Work out the finished part from the listing and answer in its coordinate system (mm). Give positions to 0.01 mm unless a question says otherwise; leave off trailing zeros. Loops run counter-clockwise (first coordinate to the right, second up) from the corner with the lowest first, then second, coordinate; pieces in that order, holes last.
```python
from build123d import *

# Parameters (mm, degrees)
EXTRUDE1_DEPTH     = 3.175
SKETCH4_R          = 3.772
EXTRUDE3_DEPTH     = 1.27
SKETCH6_R          = 3
CUT_EXTRUDE1_DEPTH = 181.936091825


with BuildPart() as part:
    # Sketch1 → Extrude1 (new body)
    with BuildSketch(Plane.XY):
        with BuildLine():
            Line((104.316218765, 133.220465896), (119.791106556, 133.220465896))
            ThreePointArc((119.791106556, 133.220465896), (122.35366266, 126.720465896), (119.791106556, 120.220465896))
            Line((119.791106556, 120.220465896), (104.316218765, 120.220465896))
            ThreePointArc((104.316218765, 120.220465896), (101.75366266, 126.720465896), (104.316218765, 133.220465896))
        make_face()
    extrude(amount=EXTRUDE1_DEPTH)

    # Sketch4 → Extrude3 (add)
    with BuildSketch(Plane.XY.offset(3.175)):
        with Locations((117.35366266, 126.720465896)):
            Circle(SKETCH4_R)
    extrude(amount=EXTRUDE3_DEPTH)

    # Sketch6 → Cut-Extrude1 (cut, through all)
    with BuildSketch(Plane(origin=(0, 0, 0), x_dir=(-1, 0, 0), z_dir=(0, 0, -1))):
        with Locations((-117.35366266, 126.720465896)):
            Circle(SKETCH6_R)
    extrude(amount=-CUT_EXTRUDE1_DEPTH, mode=Mode.SUBTRACT)


solid = part.part
```
Q1. Section D-D on x = 107.5 is taken. Give the vertices of the cut face in (y, z) (3 decimals), plus the area to 3 significant figures.
Q2. Section B-B on y = 126.25 is taken. Give the vertices of the cut face in (x, z) (3 decimals).
Q3. Section C-C on z = 1 is taken. Give the vertices of the cut face in (x, y) (3 decimals), plus the area to 3 significant figures.
Q4. Determine the mould class of faces 1 (the face through (122.353, 126.821, 1.565)), 2 (the face through (120.951, 127.853, 3.801)), 3 (the face through (112, 133.22, 2)), 4 (the face through (114.49, 127.62, 2.19)) for opening direction X: +X half, -X half, draft (parallel to the pull), parting line (faces both ways), or undercut.
Q5. Section A-A on x = 120 is taken. Give the vertices of the cut face in (y, z) (3 decimals).
Q6. Consider line 1 along Z through (x, y) = (118.25, 121.75) (3 decimals); line 2 along X through (y, z) = (128, 3.9); line 3 along Y through (x, z) = (116.5, 0.7). Determine where each line is inside the solid, lowest interval first.
Check result:
1. outline: (120.22, 0) - (133.22, 0) - (133.22, 3.175) - (120.22, 3.175) - close
1. area: 41.3 mm2
2. outline: (101.765, 0) - (114.391, 0) - (114.391, 4.445) - (113.611, 4.445) - (113.611, 3.175) - (101.765, 3.175) - close; (120.317, 0) - (122.342, 0) - (122.342, 3.175) - (121.096, 3.175) - (121.096, 4.445) - (120.317, 4.445) - close
3. outline: (104.316, 120.22) - (119.791, 120.22) arc R9.525 ccw to (119.791, 133.22) - (104.316, 133.22) arc R9.525 ccw to start; hole circle Ø6 at (117.354, 126.72)
3. area: 219 mm2
4. face 1: +X half
4. face 2: parting line
4. face 3: draft
4. face 4: undercut
5. outline: (120.452, 0) - (125.307, 0) - (125.307, 4.445) - (124.033, 4.445) - (124.033, 3.175) - (120.452, 3.175) - close; (128.134, 0) - (132.989, 0) - (132.989, 3.175) - (129.408, 3.175) - (129.408, 4.445) - (128.134, 4.445) - close
6. line 1: z = 0 to 3.175
6. line 2: x = 113.81 to 114.64, 120.07 to 120.9
6. line 3: y = 120.22 to 123.84, 129.6 to 133.22
